For this review, use the dimensioned drawing (mm, ordinates from the lowest corner) and the shaded views. A direction names the side the tool comes from. Round coordinates to 2 decimals unless told otherwise and drop trailing zeros. Write each loop counter-clockwise with the first axis right and the second up, starting at its lowest first coordinate (ties: lowest second). Pieces come first, ordered by that corner, then holes. Notation, with made-up numbers: (69, 69) -> (121, 69) arc R33 cw to (121, 107) -> close; hole circle Ø1 at (56.5, 0). An arc over 180 degrees is marked (long way). Answer as CSV lines item,"result". Start each with the question number.
Item 1: Take a section at C-C on x = 12. Give the boundary of the cut face in (y, z).
Item 2: Wall thickness on probe 1 along X at (y, z) = (6.75, 9); probe 2 along Y at (x, z) = (12.5, 7); probe 3 along Z at (x, y) = (8.5, 16.75): over which ranges is each line inside the solid? List them lowest first. Write a range as from..to.
Item 3: Take a section at D-D on z = 2. Give the boundary of the cut face in (x, y), then the cut area to 3 significant figures.
Item 4: Machinability: for the marked faces 1, 2 and 3, which of the approach directions +Z, -Z, +X, -X, +Y, -Y give a long, thin tool a straight path to every point of the face, cutting with its end or side? Answer none if there is none.
Item 5: Take a section at A-A on z = 9.5. Give the boundary of the cut face in (x, y), then the cut area to 3 significant figures.
Item 6: Take a section at B-B on y = 22.25. Give the boundary of the cut face in (x, z).
Item 7: For pin 1 Ø0.6 at (x, z) = (12.5, 8.5) entering from -Y; pin 2 Ø1.5 at (y, z) = (5, 6.5) entering from -X; pin 3 Ø0.9 at (y, z) = (6, 6.5) entering from +X, all flat-tipped, find the tip position at first contact; note any pin that passes through.
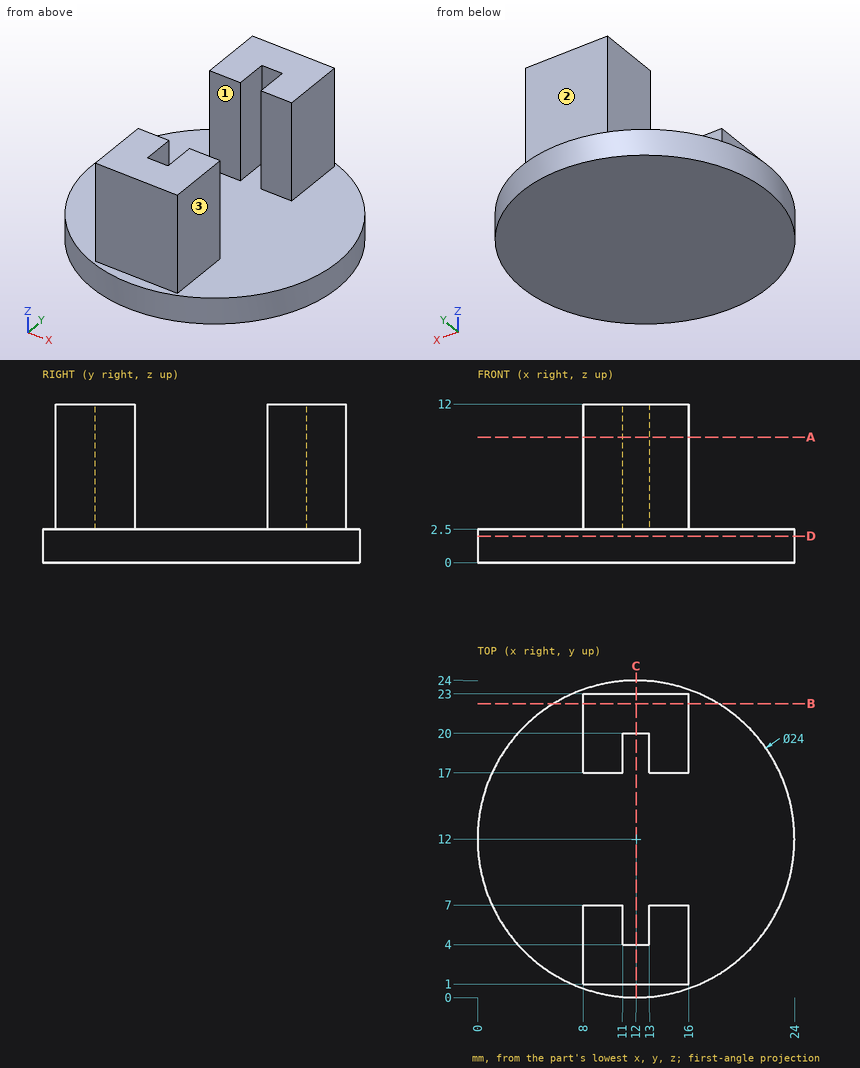
Output values:
1,outline,"(0, 0) -> (24, 0) -> (24, 2.5) -> (23, 2.5) -> (23, 12) -> (20, 12) -> (20, 2.5) -> (4, 2.5) -> (4, 12) -> (1, 12) -> (1, 2.5) -> (0, 2.5) -> close"
2,probe 1,"x = 8..11, 13..16"
2,probe 2,"y = 1..4, 20..23"
2,probe 3,"z = 0..2.5"
3,outline,"circle Ø24 at (12, 12)"
3,area,"452 mm^2"
4,face 1,"+Z, +X, -X"
4,face 2,"+Z, +X, -X, +Y"
4,face 3,"+Z, +X, +Y, -Y"
5,outline,"(8, 1) -> (16, 1) -> (16, 7) -> (13, 7) -> (13, 4) -> (11, 4) -> (11, 7) -> (8, 7) -> close; (8, 17) -> (11, 17) -> (11, 20) -> (13, 20) -> (13, 17) -> (16, 17) -> (16, 23) -> (8, 23) -> close"
5,area,"84.0 mm^2"
6,outline,"(5.76, 0) -> (18.24, 0) -> (18.24, 2.5) -> (16, 2.5) -> (16, 12) -> (8, 12) -> (8, 2.5) -> (5.76, 2.5) -> close"
7,pin 1,"stops at y = 1"
7,pin 2,"stops at x = 8"
7,pin 3,"stops at x = 16"
